Build history of the part. All positions in model axes, mm. Face numbers are marked on the shaded views. A direction names the side the tool comes from. Round coordinates to 2 decimals unless told otherwise and drop trailing zeros. Write each loop counter-clockwise with the first axis right and the second up, starting at its lowest first coordinate (ties: lowest second). Pieces come first, ordered by that corner, then holes. Notation, with made-up numbers: (-31, 4) -> (14, 4) arc R26 ccw to (14, 35) -> close; hole circle Ø9 at (24, -39). An arc over 180 degrees is marked (long way). Return JSON: item names as keys, results as strings.
from build123d import *

# Parameters (mm, degrees)
F0_W     = 101.6
F0_H     = 53.34
F1_DEPTH = 1
F3_D     = 3
F4_W     = 9.525
F4_H     = 11.43
F4_W_2   = 6.35
F4_W_3   = 11.43
F4_H_2   = 8.89
F4_W_4   = 1.905
F5_DEPTH = 11


with BuildPart() as f1:
    # F0 (on Top) → F1 (new body)
    with BuildSketch(Plane.XY):
        Rectangle(F0_W, F0_H)
    extrude(amount=F1_DEPTH)

    # F3 (through all)
    with Locations(Plane.XY.offset(1)):
        with Locations((-35.56, 24.13), (39.37, 24.13), (45.72, -24.13), (15.24, -19.05), (-36.83, -24.13)):
            Hole(F3_D / 2)

    # F4 (on face) → F5 (join)
    with BuildSketch(Plane.XY.offset(1)):
        with Locations((-46.0375, 11.43)):
            Rectangle(F4_W, F4_H)
        with Locations((-53.975, 11.43)):
            Rectangle(F4_W_2, F4_H)
        with Locations((-45.085, -19.05)):
            Rectangle(F4_W_3, F4_H_2)
        with Locations((-51.7525, -19.05)):
            Rectangle(F4_W_4, F4_H_2)
    extrude(amount=F5_DEPTH)


solid = f1.part
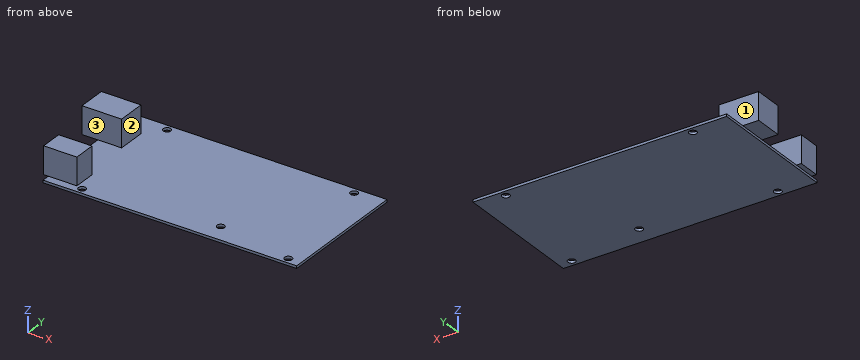
Q1. Saw through at D-D on y = -9. List the corners of the cut face in (x, z).
Verdict:
{"outline": "(-50.8, 0) -> (50.8, 0) -> (50.8, 1) -> (-50.8, 1) -> close"}
Q2. Wall check: L1, parallel to Y at x = 15.24, z = 0.45; L2, parallel to Y at x = -36.83, z = 0.3; L3, parallel to Y at x = 39.37, z = 0.4. Give the ranges that are in metal, low to high.
Verdict:
{"L1": "y = -26.67 to -20.55, -17.55 to 26.67", "L2": "y = -26.67 to -25.63, -22.63 to 23.33, 24.93 to 26.67", "L3": "y = -26.67 to 22.63, 25.63 to 26.67"}
Q3. Saw through at B-B on z = 3. List the corners of the cut face in (x, y) (3 decimals), then the cut area to 3 significant figures.
Verdict:
{"outline": "(-57.15, 5.715) -> (-41.275, 5.715) -> (-41.275, 17.145) -> (-57.15, 17.145) -> close; (-52.705, -23.495) -> (-39.37, -23.495) -> (-39.37, -14.605) -> (-52.705, -14.605) -> close", "area": "300 mm²"}
Q4. Saw through at C-C on x = -42.5. List the corners of the cut face in (y, z) (3 decimals), then the cut area to 3 significant figures.
Verdict:
{"outline": "(-26.67, 0) -> (26.67, 0) -> (26.67, 1) -> (17.145, 1) -> (17.145, 12) -> (5.715, 12) -> (5.715, 1) -> (-14.605, 1) -> (-14.605, 12) -> (-23.495, 12) -> (-23.495, 1) -> (-26.67, 1) -> close", "area": "277 mm²"}
Q5. Saw through at A-A on x = 39.37. List the corners of the cut face in (y, z), then the cut area to 3 significant figures.
Verdict:
{"outline": "(-26.67, 0) -> (22.63, 0) -> (22.63, 1) -> (-26.67, 1) -> close; (25.63, 0) -> (26.67, 0) -> (26.67, 1) -> (25.63, 1) -> close", "area": "50.3 mm²"}
Q6. 3-axis set-ups, long thin cutter, end or side, ignore diameter. For the marked faces 1, 2 and 3: which of +Z, -Z, +X, -X, +Y, -Y reach the whole face in a straight line?
Verdict:
{"face 1": "+Z, +X, -X, +Y", "face 2": "+Z, +X, +Y", "face 3": "+Z, +X, -X"}
Q7. Pin check, flat tips, straight feed: pin 1 Ø4.5 at (y, z) = (-17, 4) entering from -X (3 decimals); pin 2 Ø0.6 at (x, y) = (-52, -20) entering from -Z; pin 3 Ø5 at (x, y) = (-7, 7.5) entering from +Z; pin 4 Ø2 at (x, y) = (32.5, -18) entering from -Z. Stop position of each tip, or through.
Verdict:
{"pin 1": "stops at x = -52.705", "pin 2": "stops at z = 1", "pin 3": "stops at z = 1", "pin 4": "stops at z = 0"}
